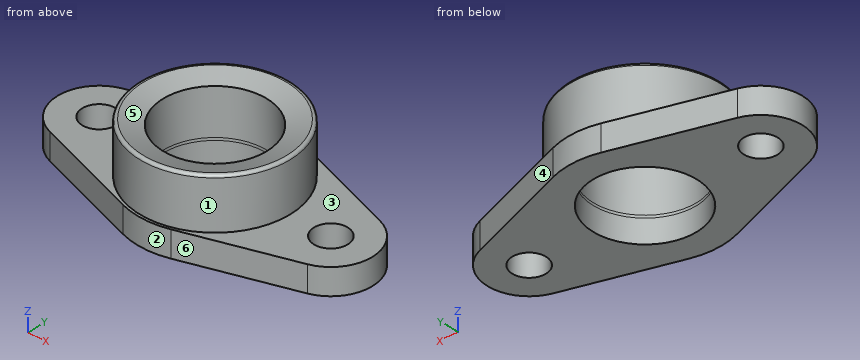
from build123d import *

# Parameters (mm, degrees)
SKETCH_R   = 20
SKETCH_R_2 = 6.5
PAD_DEPTH  = 10
FILLET_R   = 1


with BuildPart() as revolution:
    # Sketch001 → Revolution (revolve)
    with BuildSketch(Plane.XZ):
        Polygon((20, 9), (20, 27.588457), (29, 30), (29, 9), align=None)
    revolve(axis=Axis((0, 0, 0), (0, 0, 1)))


with BuildPart() as fillet_body:
    # Sketch → Pad (new body)
    with BuildSketch(Plane.XY):
        with BuildLine():
            ThreePointArc((9.333333, 28.511206), (0, 30), (-9.333333, 28.511206))
            Line((-49.977778, 15.205977), (-9.333333, 28.511206))
            ThreePointArc((-49.977778, 15.205977), (-61, 0), (-49.977778, -15.205977))
            Line((-49.977778, -15.205977), (-9.333333, -28.511206))
            ThreePointArc((-9.333333, -28.511206), (0, -30), (9.333333, -28.511206))
            Line((9.333333, -28.511206), (49.977778, -15.205977))
            ThreePointArc((49.977778, -15.205977), (61, 0), (49.977778, 15.205977))
            Line((9.333333, 28.511206), (49.977778, 15.205977))
        make_face()
        Circle(SKETCH_R, mode=Mode.SUBTRACT)
        with Locations((-45, 0)):
            Circle(SKETCH_R_2, mode=Mode.SUBTRACT)
        with Locations((45, 0)):
            Circle(SKETCH_R_2, mode=Mode.SUBTRACT)
    extrude(amount=PAD_DEPTH)

    # Fusion: union Revolution
    add(revolution.part)

    # Fillet
    fillet_edges = [fillet_body.edges().sort_by_distance(p)[0] for p in [
        (-29, 0, 30),
    ]]
    fillet(fillet_edges, radius=FILLET_R)


solid = fillet_body.part
Part model, mm, in its own coordinate system. Face numbers are marked on the shaded views. A direction names the side the tool comes from. Coordinates: 2 decimals unless noted, no trailing zeros. Write each loop counter-clockwise with the first axis right and the second up, starting at its lowest first coordinate (ties: lowest second). Pieces come first, ordered by that corner, then holes. Notation, with made-up numbers: M -8,61 L 5,61 A17 cw 5,74 Z; hole C 83,62 d5. An arc over 180 degrees is marked long. Return JSON: item names as keys, results as strings.
1. Saw through at C-C, the plane y = 0. Count the separate pieces of the cut face and the enclosed holes in it, then the cut area to 3 significant figures.
Determined:
{"separate pieces": "4", "enclosed holes": "0", "area": "898 mm²"}
2. Probe L1, parallel to X at y = 1, z = 6.25; L2, parallel to Z at x = 30.5, y = -19; L3, parallel to X at y = 1.5, z = 12.5. List the from-to ranges inside material, lowest first.
Determined:
{"L1": "-60.97 to -51.42, -38.58 to -19.97, 19.97 to 38.58, 51.42 to 60.97", "L2": "0 to 10", "L3": "-28.96 to -19.94, 19.94 to 28.96"}
3. 3-axis set-ups, long thin cutter, end or side, ignore diameter. For the marked faces 1 and 2: which of +Z, -Z, +X, -X, +Y, -Y reach the whole face in a straight line?
Determined:
{"face 1": "+Z", "face 2": "+Z, -Z, -Y"}
4. Flat gauge pins, fed straight in: pin 1 Ø8 at (x, z) = (28, 7.5) entering from +Y; pin 2 Ø21 at (x, y) = (45, 0) entering from +Z; pin 3 Ø12 at (x, z) = (42.5, 5.5) entering from -Y; pin 4 Ø10 at (x, y) = (10, 23) entering from +Z. Where does each tip first touch, or does it go through?
Determined:
{"pin 1": "y = 23.71", "pin 2": "z = 10", "pin 3": "y = -19.62", "pin 4": "z = 29.7"}
5. Saw through at B-B, the plane z = 15.75. Write the cut outline in (x, y), then the cut area to 3 significant figures.
Determined:
{"outline": "C 0,0 d58; hole C 0,0 d40", "area": "1,390 mm²"}
6. Pull direction Y, two halves, no side cores. Call the marked faces 3, 4, 5 and 6: pulls with the +Y half, pulls with the -Y half, needs draft (parallel to the pull), parting line crosses it, or undercut.
Determined:
{"face 3": "needs draft", "face 4": "pulls with the +Y half", "face 5": "undercut", "face 6": "pulls with the -Y half"}
7. Saw through at A-A, the plane x = 45. Write the cut outline in (y, z), then the cut area to 3 significant figures.
Determined:
{"outline": "M -16.84,0 L -6.5,0 L -6.5,10 L -16.84,10 Z; M 6.5,0 L 16.84,0 L 16.84,10 L 6.5,10 Z", "area": "207 mm²"}
8. Saw through at D-D, the plane x = -42.5. Write the cut outline in (y, z), then the cut area to 3 significant figures.
Determined:
{"outline": "M -17.65,0 L -6,0 L -6,10 L -17.65,10 Z; M 6,0 L 17.65,0 L 17.65,10 L 6,10 Z", "area": "233 mm²"}
